Autodesk Inventor part; units mm, degrees
ref_plane "YZ Plane" through (0, 0, 0) normal (1, 0, 0) x (0, 1, 0)
ref_plane "XZ Plane" through (0, 0, 0) normal (0, 1, 0) x (-1, 0, 0)
ref_plane "XY Plane" through (0, 0, 0) normal (0, 0, 1) x (1, 0, 0)
sketch "Sketch1" plane through (0, 0, 0) normal (0, 1, 0) x (-1, 0, 0)
  line L0 (20, 20) -> (-20, 20)
  line L1 (-20, 20) -> (-20, -20)
  line L2 (-20, -20) -> (20, -20)
  line L3 (20, -20) -> (20, 20)
  line L4 (20, 20) -> (-20, -20) construction
  line L5 (-20, 20) -> (20, -20) construction
  line L6 (16, 16) -> (-16, 16)
  line L7 (-16, 16) -> (-16, -16)
  line L8 (-16, -16) -> (16, -16)
  line L9 (16, -16) -> (16, 16)
  line L10 (16, 16) -> (-16, -16) construction
  line L11 (-16, 16) -> (16, -16) construction
  point P0 (0, 0)
  dimension "d0" = 40
  dimension "d1" = 40
  dimension "d2" = 32
  dimension "d3" = 32
extrude "Extrusion1" add sketch "Sketch1" along normal blind 5 contours L3 L2 L1 L0 | L9 L8 L7 L6
sketch "Sketch2" plane through (0, 5, 0) normal (0, 1, 0) x (1, 0, 0)
  circle A0 centre (0, 0) radius 15
  dimension "d7" = 30
extrude "Extrusion2" add sketch "Sketch2" along normal blind 2.5
sketch "Sketch3" plane through (0, 0, 0) normal (0, -1, 0) x (1, 0, 0)
  circle A0 centre (0, 0) radius 19
  dimension "d10" = 38
extrude "Extrusion3" add sketch "Sketch3" along normal blind 95
fillet "Fillet1" radius 2.5 1 edges at (-19, -95, 0)
fillet "Fillet2" radius 2 4 edges at (20, 2.5, -20) (-20, 2.5, -20) (-20, 2.5, 20) (20, 2.5, 20)
hole "Hole1" at (16, 0, -16) at (16, 0, 16) at (-16, 0, -16) at (-16, 0, 16) direction (0, 1, 0) diameter 3 depth 5 tip angle 118
sketch "Sketch4" plane through (0, 7.5, 0) normal (0, 1, 0) x (1, 0, 0)
  circle A0 centre (0, 0) radius 3
  dimension "d22" = 6
extrude "Extrusion4" add sketch "Sketch4" along normal blind 25
equation "\"d1\" = d0"
equation "\"d3\" = d2"
properties part number "Nanotec-DH052-120E-Servo"
Here's how the part is built. I have some questions about the finished solid (model axes, mm). A direction names the side the tool comes from. Coordinates: 2 decimals unless noted, no trailing zeros. Order: outer loops, then holes, each group sorted by start corner. A loop starts at its lowest first (then second) coordinate and runs counter-clockwise, first axis right, second up. Notation, with made-up numbers: M -38,30 L 21,30 A22 cw 21,64 Z; hole C 2,43 d3. An arc over 180 degrees is marked long. Answer as CSV lines item,"result".
Item 1: Imagine slicing it at C-C on y = -40. Write out the boundary of the cut face in (x, z), plus the area to 3 significant figures.
Results found:
outline,"C 0,0 d38"
area,"1,130 mm2"
Item 2: For pin 1 (3.5 mm diameter, centred on x = 16, z = -16, fed in from -Y); pin 2 (8 mm diameter, centred on x = -5, y = -46, fed in from -Z); pin 3 (6 mm diameter, centred on y = -47, z = 14, fed in from -X); pin 4 (1.8 mm diameter, centred on x = 16, z = 16, fed in from -Y), each with a flat end and sliding along its axis, tell me the tip position at first contact or that it passes through.
Results found:
pin 1,"y = 0"
pin 2,"z = -18.97"
pin 3,"x = -15.49"
pin 4,"through"
Item 3: Imagine slicing it at B-B on y = 22.5. Write out the boundary of the cut face in (x, z), plus the area to 3 significant figures.
Results found:
outline,"C 0,0 d6"
area,"28.3 mm2"
Item 4: Imagine slicing it at A-A on x = 0. Write out the boundary of the cut face in (y, z).
Results found:
outline,"M -95,-16.5 A2.5 ccw -92.5,-19 L 0,-19 L 0,-20 L 5,-20 L 5,-15 L 7.5,-15 L 7.5,-3 L 32.5,-3 L 32.5,3 L 7.5,3 L 7.5,15 L 5,15 L 5,20 L 0,20 L 0,19 L -92.5,19 A2.5 ccw -95,16.5 Z"
Item 5: If I drill on line 1 (X direction, y = 1, z = 16); line 2 (Y direction, x = 7, z = -15), over which ranges is the centre line in solid material (lowest first)?
Results found:
line 1,"-20 to -17.5, -14.5 to 14.5, 17.5 to 20"
line 2,"-95 to 5"
Item 6: We'd pull the mould along X, two halves only. Please class faces 4 (the face through (20, 2, 0)), 5 (the face through (15.93, 2.54, -14.5)), 6 (the face through (-3, 20, 0)): +X half, -X half, draft (parallel to the pull), parting line (faces both ways), or undercut.
Results found:
face 4,"+X half"
face 5,"undercut"
face 6,"parting line"
Item 7: On a 3-axis mill with a long thin cutter (end or side, diameter ignored), from which of +Z, -Z, +X, -X, +Y, -Y can I reach the whole of each face in a straight line? I mean faces 1 (the face through (-9, 5, 14)), 2 (the face through (8.767, -45.602, 16.856)), 3 (the face through (0, 32.5, 0)). Say none if no direction works.
Results found:
face 1,"+Y"
face 2,"-Y"
face 3,"+Z, -Z, +X, -X, +Y"
